Autodesk Inventor part; units mm, degrees
ref_plane "YZ Plane" through (0, 0, 0) normal (1, 0, 0) x (0, 1, 0)
ref_plane "XZ Plane" through (0, 0, 0) normal (0, 1, 0) x (-1, 0, 0)
ref_plane "XY Plane" through (0, 0, 0) normal (0, 0, 1) x (1, 0, 0)
sketch "Sketch1" plane through (0, 0, 0) normal (0, 0, 1) x (1, 0, 0)
  circle A0 centre (0, 0) radius 2.5
  circle A1 centre (0, 0) radius 5
  line L0 (-1.7678, -1.7678) -> (-12.3744, 8.8388)
  line L1 (-12.3744, 8.8388) -> (-15.9099, 5.3033)
  line L2 (-15.9099, 5.3033) -> (5, -15.6066)
  line L3 (5, -15.6066) -> (5, -22.6777)
  line L4 (5, -22.6777) -> (1.4645, -26.2132)
  line L5 (-5.6066, -26.2132) -> (-16.2132, -15.6066)
  line L6 (1.7678, 1.7678) -> (-8.8388, 12.3744)
  line L7 (-15.9099, 12.3744) -> (-19.4454, 8.8388)
  line L8 (-19.4454, 8.8388) -> (-19.4454, 1.7678)
  line L9 (-19.4454, 1.7678) -> (1.4645, -19.1421)
  line L10 (1.4645, -19.1421) -> (-2.0711, -22.6777)
  line L11 (-2.0711, -22.6777) -> (-12.6777, -12.0711)
  line L12 (-12.6777, -12.0711) -> (-16.2132, -15.6066)
  line L13 (-1.7678, -1.7678) -> (1.7678, 1.7678)
  circle A2 centre (-14.4454, -13.8388) radius 2.5
  circle A3 centre (-14.4454, -13.8388) radius 5
  line L14 (-15.9099, 12.3744) -> (-8.8388, 12.3744)
  line L15 (-5.6066, -26.2132) -> (1.4645, -26.2132)
  dimension "d0" = 5
  dimension "d1" = 10
  dimension "d3" = 90
  dimension "d6" = 135
  dimension "d7" = 135
  dimension "d8" = 90
  dimension "d9" = 5
  dimension "d12" = 10
  dimension "d13" = 15
  dimension "d14" = 15
  dimension "d31" = 7.0711
  dimension "d32" = 15
  dimension "d33" = 7.0711
  dimension "d34" = 15
  dimension "d35" = 7.0711
  dimension "d36" = 7.0711
  dimension "d37" = 5
  dimension "d38" = 90
  dimension "d39" = 135
  dimension "d40" = 5
  dimension "d41" = 5
extrude "Extrusion10" add sketch "Sketch1" along normal blind 10 contours A0 L6 A1 L0 | A0 L0 A1 L6 | A1 L0 L1 L2 L3 L4 L15 L5 A3 L11 L10 L9 L8 L7 L14 L6 | A3 L5 A2 L11 | L11 A2 L5 A3 | A2 L12 picked at (-13.4317, -14.7545)
sketch "Sketch6" plane through (0, 0, 10) normal (0, 0, 1) x (1, 0, 0)
  line L0 (-1.2941, 4.8296) -> (-8.8388, 12.3744)
  line L1 (-8.8388, 12.3744) -> (-15.9099, 12.3744)
  line L2 (-15.9099, 12.3744) -> (-19.4454, 8.8388)
  line L3 (-19.4454, 8.8388) -> (-19.4454, 1.7678)
  line L4 (-19.4454, 1.7678) -> (1.4645, -19.1421)
  line L5 (1.4645, -19.1421) -> (-2.0711, -22.6777)
  line L6 (-2.0711, -22.6777) -> (-9.6158, -15.1329)
  arc A0 (-9.6158, -15.1329) -> (-13.1513, -18.6685) centre (-14.4454, -13.8388) ccw
  line L7 (-13.1513, -18.6685) -> (-5.6066, -26.2132)
  line L8 (-5.6066, -26.2132) -> (1.4645, -26.2132)
  line L9 (1.4645, -26.2132) -> (5, -22.6777)
  line L10 (5, -22.6777) -> (5, -15.6066)
  line L11 (5, -15.6066) -> (-15.9099, 5.3033)
  line L12 (-15.9099, 5.3033) -> (-12.3744, 8.8388)
  line L13 (-12.3744, 8.8388) -> (-4.8296, 1.2941)
  arc A1 (-4.8296, 1.2941) -> (-1.2941, 4.8296) centre (0, 0) ccw
  line L14 (-16.2132, -15.6066) -> (-12.6777, -12.0711)
  arc A2 (-12.6777, -12.0711) -> (-16.2132, -15.6066) centre (-14.4454, -13.8388) ccw
  circle A3 centre (0, 0) radius 2.5
  circle A4 centre (-14.4454, -13.8388) radius 2.5
extrude "Extrusion11" cut sketch "Sketch6" against normal blind 10 contours L14 A4
equation "\"d1\" = 2 * d0"
equation "\"d9\" = d0"
equation "\"d12\" = d1"
equation "\"d13\" = 3 * d0"
equation "\"d14\" = d13"
properties part number "Sawaiz Logo Ribbon 4"
Here's how the part is built. I have some questions about the finished solid (model axes, mm). A direction names the side the tool comes from. Round coordinates to 2 decimals unless told otherwise and drop trailing zeros. Order: outer loops, then holes, each group sorted by start corner. A loop starts at its lowest first (then second) coordinate and runs counter-clockwise, first axis right, second up. Notation, with made-up numbers: (-24, -7) -> (31, -7) arc R26 ccw to (31, 11) -> close; hole circle Ø5 at (87.5, -15). An arc over 180 degrees is marked (long way). Use CSV: the item, a comma, the result in double quotes.
1. I need wall thicknesses on line 1 along Y through (x, z) = (0, 5); line 2 along Y through (x, z) = (-11.25, 6); line 3 along Y through (x, z) = (-15, 5). Which ranges of each line are inside material? Lowest first, please.
Recorded:
line 1,"y = -26.21 to -20.61, -17.68 to -10.61, -5 to -2.5, 2.5 to 5"
line 2,"y = -20.57 to -9.99, -6.43 to 0.64, 7.71 to 12.37"
line 3,"y = -18.81 to -16.28, -11.4 to -8.87, -2.68 to 4.39, 6.21 to 12.37"
2. Thinking about a two-plate mould opening in X: for faces 1 (the face through (-17.653, 10.631, 4.93)), 2 (the face through (-14.117, 7.096, 4.93)), 3 (the face through (3.26, -24.42, 4.93)), 4 (the face through (-7, -7, 0)), which applies, pulls with the +X half, pulls with the -X half, needs draft (parallel to the pull), parting line crosses it, or undercut?
Recorded:
face 1,"pulls with the -X half"
face 2,"undercut"
face 3,"pulls with the +X half"
face 4,"needs draft"
3. I want a section at A-A on z = 1.25. List the corners of the cut face in (x, y) for me, and give its area (3 significant figures).
Recorded:
outline,"(-19.45, 1.77) -> (1.46, -19.14) -> (-2.07, -22.68) -> (-9.62, -15.13) arc R5 ccw (long way) to (-13.15, -18.67) -> (-5.61, -26.21) -> (1.46, -26.21) -> (5, -22.68) -> (5, -15.61) -> (-15.91, 5.3) -> (-12.37, 8.84) -> (-4.83, 1.29) arc R5 ccw (long way) to (-1.29, 4.83) -> (-8.84, 12.37) -> (-15.91, 12.37) -> (-19.45, 8.84) -> close; hole circle Ø5 at (-14.45, -13.84); hole circle Ø5 at (0, 0)"
area,"468 mm2"
4. I want a section at D-D on x = 3. List the corners of the cut face in (y, z) for me, and give its area (3 significant figures).
Recorded:
outline,"(-24.68, 0) -> (-13.61, 0) -> (-13.61, 10) -> (-24.68, 10) -> close; (-4, 0) -> (4, 0) -> (4, 10) -> (-4, 10) -> close"
area,"191 mm2"
5. I want a section at C-C on y = 0. List the corners of the cut face in (x, z) for me, and give its area (3 significant figures).
Recorded:
outline,"(-17.68, 0) -> (-10.61, 0) -> (-10.61, 10) -> (-17.68, 10) -> close; (-5, 0) -> (-2.5, 0) -> (-2.5, 10) -> (-5, 10) -> close; (2.5, 0) -> (5, 0) -> (5, 10) -> (2.5, 10) -> close"
area,"121 mm2"
6. Which directions (+Z, -Z, +X, -X, +Y, -Y) give clear straight access to the entire face, cutting with the end or side of a thin tool? Please do faces 5 (the face through (-7, -7, 10)), 6 (the face through (-0.279, -20.885, 4.93)).
Recorded:
face 5,"+Z, +X, -X, +Y, -Y"
face 6,"+Z, -Z"
7. I want a section at B-B on x = 0. List the corners of the cut face in (y, z) for me, and give its area (3 significant figures).
Recorded:
outline,"(-26.21, 0) -> (-20.61, 0) -> (-20.61, 10) -> (-26.21, 10) -> close; (-17.68, 0) -> (-10.61, 0) -> (-10.61, 10) -> (-17.68, 10) -> close; (-5, 0) -> (-2.5, 0) -> (-2.5, 10) -> (-5, 10) -> close; (2.5, 0) -> (5, 0) -> (5, 10) -> (2.5, 10) -> close"
area,"177 mm2"
8. I'm going to push flat-ended pins straight in: P1, Ø4, axis at x = -14.45, y = -13.84, coming from the +Z side; P2, Ø1.5, axis at x = -12, z = 2, coming from the -Y side; P3, Ø5, axis at x = -1.5, y = -9, coming from the -Z side; P4, Ø4, axis at x = -11.5, z = 8.5, coming from the -Y side. Where does each tip first touch, or does it pass through?
Recorded:
P1,"passes through"
P2,"stops at y = -20.57"
P3,"stops at z = 0"
P4,"stops at y = -22.32"
